Check sheet for the modelled part. Datum: model origin and axes. Units: mm. A direction names the side the tool comes from. Round coordinates to 2 decimals unless told otherwise and drop trailing zeros. Order: outer loops, then holes, each group sorted by start corner. A loop starts at its lowest first (then second) coordinate and runs counter-clockwise, first axis right, second up. Notation, with made-up numbers: (84.25, 28) -> (137.25, 28) arc R16 ccw to (137.25, 32) -> close; hole circle Ø9 at (7.25, 66.25). An arc over 180 degrees is marked (long way). Answer in a Markdown table with one row per item.
```python
from build123d import *

# Parameters (mm, degrees)
CYLINDER018_R     = 3.4
CYLINDER018_DEPTH = 44
CYLINDER017_R     = 5
CYLINDER017_DEPTH = 9
PAD006_DEPTH      = 5
PAD004_DEPTH      = 21


with BuildPart() as cylinder018:
    # Cylinder018 → Cylinder018 (new body)
    with BuildSketch(Plane(origin=(10.5, -10.1, -9), x_dir=(1, 0, 0), z_dir=(0, 0, 1))):
        Circle(CYLINDER018_R)
    extrude(amount=CYLINDER018_DEPTH)


with BuildPart() as cylinder017:
    # Cylinder017 → Cylinder017 (new body)
    with BuildSketch(Plane(origin=(10.5, -10.1, 44), x_dir=(1, 0, 0), z_dir=(0, 0, 1))):
        Circle(CYLINDER017_R)
    extrude(amount=CYLINDER017_DEPTH)


with BuildPart() as fusion014:
    # Sketch006 → Pad006 (new body)
    with BuildSketch(Plane.XY):
        with BuildLine():
            Line((-4.25, 3.75), (-4.25, 9.25))
            Line((-4.25, 9.25), (-2.65, 17.292388))
            ThreePointArc((2.65, 17.292388), (0, 20), (-2.65, 17.292388))
            Line((2.65, 17.292388), (4.25, 9.25))
            Line((4.25, 3.75), (4.25, 9.25))
            ThreePointArc((4.25, -3.75), (5.657274, 0), (4.25, 3.75))
            Line((4.25, -3.75), (4.25, -9.25))
            Line((2.65, -17.292388), (4.25, -9.25))
            ThreePointArc((-2.65, -17.292388), (0, -20), (2.65, -17.292388))
            Line((-4.25, -9.25), (-2.65, -17.292388))
            Line((-4.25, -3.75), (-4.25, -9.25))
            ThreePointArc((-4.25, 3.75), (-5.657274, 0), (-4.25, -3.75))
        make_face()
    extrude(amount=PAD006_DEPTH)


with BuildPart() as fusion014_1:
    # Body006 placement: moved
    add(fusion014.part.moved(Location((10.5, -10, 48))))

    # Fusion014: union Cylinder017
    add(cylinder017.part)


with BuildPart() as obj1:
    # Sketch004 → Pad004 (new body)
    with BuildSketch(Plane.YZ):
        Polygon((-33, -0.5), (0, -0.5), (0, -5.5), (-38, -5.5), (-38, 50.5), (0, 50.5), (0, 45.5), (-33, 45.5), align=None)
    extrude(amount=PAD004_DEPTH)

    # Cut008: cut Fusion014
    add(fusion014_1.part, mode=Mode.SUBTRACT)

    # Cut009: cut Cylinder018
    add(cylinder018.part, mode=Mode.SUBTRACT)


solid = obj1.part
```
(1) Tool access check on faces 1 (the flat face through (6.25, -16, 49)), 2 (the cylindrical face through (13.743, -9.079, -3.035)), 3 (the flat face through (10, -16, 45.5)). Record the directions out of +Z, -Z, +X, -X, +Y, -Y that give a thin tool (end or side, any length) a straight path to the whole face; none if there is none.
Solutions:
| item | result |
|---|---|
| face 1 | +Z |
| face 2 | +Z, -Z |
| face 3 | +X, -X, +Y |
(2) Section check A-A on x = 10.5. Record the boundary of the cut face in (y, z).
Solutions:
| item | result |
|---|---|
| outline | (-38, -5.5) -> (-13.5, -5.5) -> (-13.5, -0.5) -> (-33, -0.5) -> (-33, 45.5) -> (-15.1, 45.5) -> (-15.1, 48) -> (-30, 48) -> (-30, 50.5) -> (-38, 50.5) -> close; (-6.7, -5.5) -> (0, -5.5) -> (0, -0.5) -> (-6.7, -0.5) -> close; (-5.1, 45.5) -> (0, 45.5) -> (0, 48) -> (-5.1, 48) -> close |
(3) Section check C-C on y = -10.1. Record the boundary of the cut face in (x, z), plus the area to 3 significant figures.
Solutions:
| item | result |
|---|---|
| outline | (0, -5.5) -> (7.1, -5.5) -> (7.1, -0.5) -> (0, -0.5) -> close; (0, 45.5) -> (5.5, 45.5) -> (5.5, 48) -> (4.84, 48) -> (4.84, 50.5) -> (0, 50.5) -> close; (13.9, -5.5) -> (21, -5.5) -> (21, -0.5) -> (13.9, -0.5) -> close; (15.5, 45.5) -> (21, 45.5) -> (21, 50.5) -> (16.16, 50.5) -> (16.16, 48) -> (15.5, 48) -> close |
| area | 123 mm^2 |
(4) Section check B-B on y = -31. Record the boundary of the cut face in (x, z).
Solutions:
| item | result |
|---|---|
| outline | (0, -5.5) -> (21, -5.5) -> (21, -0.5) -> (0, -0.5) -> close; (0, 45.5) -> (21, 45.5) -> (21, 50.5) -> (0, 50.5) -> close |
(5) Scan lines: probe 1 along Z at (x, y) = (13.5, -29); probe 2 along Y at (x, z) = (10.5, -4.5); probe 3 along Y at (x, z) = (10.5, 46.85). Record each from-to range of solid material in increasing order. Write a range as from..to.
Solutions:
| item | result |
|---|---|
| probe 1 | -5.5..-0.5, 45.5..50.5 |
| probe 2 | -38..-13.5, -6.7..0 |
| probe 3 | -38..-15.1, -5.1..0 |
(6) Draft check along X on faces 4 (the flat face through (10, -17, -0.5)), 5 (the flat face through (21, -34, 25)), 6 (the flat face through (14.75, -16, 49)). Enter one of: pulls with the +X half, pulls with the -X half, needs draft (parallel to the pull), parting line crosses it, or undercut.
Solutions:
| item | result |
|---|---|
| face 4 | needs draft |
| face 5 | pulls with the +X half |
| face 6 | undercut |
(7) Section check D-D on z = 41.5. Record the boundary of the cut face in (x, y).
Solutions:
| item | result |
|---|---|
| outline | (0, -38) -> (21, -38) -> (21, -33) -> (0, -33) -> close |
(8) Depth check by flat-ended pin: pin 1 Ø8 at (x, z) = (14.5, 33.5) entering from +Y; pin 2 Ø11 at (x, y) = (10.5, -10.1) entering from +Z. Enter the tip coordinate at first touch or a pass-through.
Solutions:
| item | result |
|---|---|
| pin 1 | y = -33 |
| pin 2 | z = 48 |
